from build123d import *

# Parameters (mm, degrees)
SKETCH1_R           = 2.55
BOSS_EXTRUDE1_DEPTH = 10
SKETCH2_R           = 1.5
CUT_EXTRUDE1_DEPTH  = 5
FILLET1_R           = 2
FILLET2_R           = 2


with BuildPart() as part:
    # Sketch1 → Boss-Extrude1 (new body)
    with BuildSketch(Plane.XY):
        Polygon((-21.861045086, 19.601121192), (-11.861045086, 19.601121192), (18.138954914, -20.678878808), (48.138954914, -20.678878808), (48.138954914, -25.678878808), (-81.861045086, -25.678878808), (-81.861045086, -20.678878808), (-51.861045086, -20.678878808), align=None)
        with Locations((-16.861045086, 14.601121192)):
            Circle(SKETCH1_R, mode=Mode.SUBTRACT)
        Polygon((-41.861045086, -20.678878808), (-21.861045086, 9.601121192), (-21.861045086, -20.678878808), align=None, mode=Mode.SUBTRACT)
        Polygon((-11.861045086, 9.601121192), (-11.861045086, -20.678878808), (8.138954914, -20.678878808), align=None, mode=Mode.SUBTRACT)
    extrude(amount=BOSS_EXTRUDE1_DEPTH)

    # Sketch2 → Cut-Extrude1 (cut)
    with BuildSketch(Plane(origin=(0, -20.678878808, 0), x_dir=(1, 0, 0), z_dir=(0, 1, 0))):
        with Locations(Location((43.138954914, -5, 0), (0, 0, 180))):
            Circle(SKETCH2_R)
        with Locations(Location((-76.861045086, -5, 0), (0, 0, 180))):
            Circle(SKETCH2_R)
    extrude(amount=-CUT_EXTRUDE1_DEPTH, mode=Mode.SUBTRACT)

    # Fillet1
    fillet1_edges = [part.edges().sort_by_distance(p)[0] for p in [
        (-21.861045086, 19.601121192, 5),
        (-11.861045086, 19.601121192, 5),
        (18.138954914, -20.678878808, 5),
        (-51.861045086, -20.678878808, 5),
        (-41.861045086, -20.678878808, 5),
        (-21.861045086, -20.678878808, 5),
        (-21.861045086, 9.601121192, 5),
        (8.138954914, -20.678878808, 5),
        (-11.861045086, 9.601121192, 5),
        (-11.861045086, -20.678878808, 5),
    ]]
    fillet(fillet1_edges, radius=FILLET1_R)

    # Fillet2
    fillet2_edges = [part.edges().sort_by_distance(p)[0] for p in [
        (-16.861045086, -25.678878808, 10),
        (33.641047291, -20.678878808, 10),
        (-31.002101255, -20.678878808, 0),
        (-31.002101255, -20.678878808, 10),
        (-21.861045086, -7.867319769, 0),
        (-21.861045086, -7.867319769, 10),
        (-32.670934833, -6.765051884, 0),
        (-32.670934833, -6.765051884, 10),
        (-11.861045086, -7.867319769, 0),
        (-11.861045086, -7.867319769, 10),
        (-2.719988918, -20.678878808, 0),
        (-2.719988918, -20.678878808, 10),
        (-1.05115534, -6.765051884, 0),
        (-1.05115534, -6.765051884, 10),
        (-67.363137464, -20.678878808, 0),
        (-67.363137464, -20.678878808, 10),
        (-36.861045086, -0.538878808, 0),
        (-36.861045086, -0.538878808, 10),
        (3.138954914, -0.538878808, 0),
        (3.138954914, -0.538878808, 10),
        (-16.861045086, 19.601121192, 0),
        (-11.967812043, 19.388477142, 0),
        (-21.75427813, 19.388477142, 0),
        (-16.861045086, 19.601121192, 10),
        (-11.967812043, 19.388477142, 10),
        (-21.75427813, 19.388477142, 10),
        (-22.446831524, -20.093092371, 0),
        (-22.446831524, -20.093092371, 10),
        (-23.285574477, 4.859659218, 0),
        (33.641047291, -20.678878808, 0),
        (-23.285574477, 4.859659218, 10),
        (-39.904483028, -19.626366072, 0),
        (-39.904483028, -19.626366072, 10),
        (-11.275258649, -20.093092371, 0),
        (-11.275258649, -20.093092371, 10),
        (-10.436515696, 4.859659218, 0),
        (-10.436515696, 4.859659218, 10),
        (6.182392855, -19.626366072, 0),
        (6.182392855, -19.626366072, 10),
        (-51.967812043, -20.466234759, 0),
        (-51.967812043, -20.466234759, 10),
        (18.24572187, -20.466234759, 0),
        (18.24572187, -20.466234759, 10),
        (-16.861045086, -25.678878808, 0),
    ]]
    fillet(fillet2_edges, radius=FILLET2_R)


solid = part.part
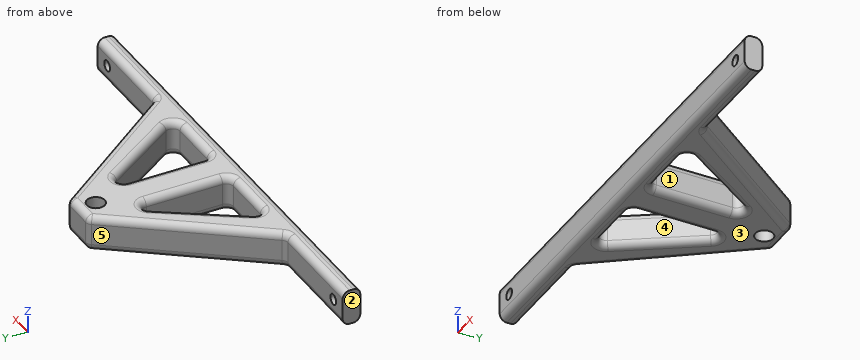
Could you check a few things on this model? Use its own coordinates, in mm. Face numbers are marked on the shaded views. A direction names the side the tool comes from. Round coordinates to 2 decimals unless told otherwise and drop trailing zeros. Order: outer loops, then holes, each group sorted by start corner. A loop starts at its lowest first (then second) coordinate and runs counter-clockwise, first axis right, second up.
(1) Imagine slicing it at A-A (x = 20.5). Write out the boundary of the cut face in (y, z), plus the area to 3 significant figures.
Response values:
outline: (-25.68, 2) arc R2 ccw to (-23.68, 0) - (-22.68, 0) arc R2 ccw to (-20.68, 2) - (-20.68, 8) arc R2 ccw to (-22.68, 10) - (-23.68, 10) arc R2 ccw to (-25.68, 8) - close
area: 46.6 mm2
(2) I'm going to push flat-ended pins straight in: pin 1 (3 mm diameter, centred on x = -74.5, z = 4.5, fed in from +Y); pin 2 (5 mm diameter, centred on y = -12, z = 6, fed in from +X); pin 3 (1 mm diameter, centred on y = 3, z = 1, fed in from +X). Where does each tip first touch, or does it pass through?
Response values:
pin 1: stops at y = -20.68
pin 2: stops at x = 13.54
pin 3: stops at x = 0.64
(3) Please list where these lines run through material, in increasing order: line 1 along X through (y, z) = (-23, 4); line 2 along X through (y, z) = (-15.5, 5.75); line 3 along Y through (x, z) = (19.5, 7.5).
Response values:
line 1: x = -81.86 to -77.98, -75.74 to 42.02, 44.26 to 48.14
line 2: x = -48 to -38.44, -21.86 to -11.86, 4.72 to 14.28
line 3: y = -25.68 to -20.68
(4) Imagine slicing it at B-B (z = 5). Count the separate pieces of the cut face and the enclosed holes in it, plus the area to 3 significant figures.
Response values:
separate pieces: 3
enclosed holes: 3
area: 1,630 mm2
(5) If we mould it in two halves opening along X, with no side actions, what happens to the marked faces 3, 4 and 5? For each: released by +X, released by -X, zero draft, split by the parting line, or undercut.
Response values:
face 3: zero draft
face 4: undercut
face 5: released by -X
(6) Which directions (+Z, -Z, +X, -X, +Y, -Y) give clear straight access to the entire face, cutting with the end or side of a thin tool? Please do the marked faces 1 and 2.
Response values:
face 1: +Z, -Z
face 2: +Z, -Z, -X, +Y, -Y
